from build123d import *

# Parameters (mm, degrees)
PAD_DEPTH    = 180
PAD001_DEPTH = 180


with BuildPart() as part:
    # Sketch → Pad (new body)
    with BuildSketch(Plane.XZ):
        Polygon((1.709151, 14), (0.847738, 14), (0.847738, 15), (2.609062, 15), (2.609062, 12.991093), (1, 11.170912), (1, 1.090989), (14, 1.090989), (14, 11.170912), (12.390938, 12.991093), (12.390938, 15), (14.152262, 15), (14.152262, 14), (13.290849, 14), (13.290849, 13.145577), (15, 11.212176), (15, 0), (0, 0), (0, 11.212176), (1.709151, 13.145577), align=None)
    extrude(amount=PAD_DEPTH)

    # Sketch001 → Pad001 (join)
    with BuildSketch(Plane.XZ):
        Polygon((1.670899, 13.98237), (0.833981, 13.98237), (0.833981, 15.0478), (14.219909, 15.0478), (14.219909, 13.970164), (13.277989, 13.970164), (13.277989, 13.140446), (14.96773, 13.140446), (14.96773, 15.855778), (0.035527, 15.855778), (0.035527, 13.198529), (1.670899, 13.198529), align=None)
    extrude(amount=PAD001_DEPTH)


solid = part.part
Work out the finished part from the listing and answer in its coordinate system (mm). A direction names the side the tool comes from. Give positions to 0.01 mm unless a question says otherwise; leave off trailing zeros. Order: outer loops, then holes, each group sorted by start corner. A loop starts at its lowest first (then second) coordinate and runs counter-clockwise, first axis right, second up. Notation, with made-up numbers: (18.5, 24) -> (50.5, 24) arc R6 cw to (50.5, 34) -> close; hole circle Ø3 at (12, 47.5). An arc over 180 degrees is marked (long way). Answer as a JSON object with one key per item and string values. Group by question number.
1. Section B-B on z = 7.5 is taken. Determine the outline of the cut face in (x, y).
2. Consider line 1 along X through (y, z) = (-63, 10); line 2 along Z through (x, y) = (5.75, -39); line 3 along X through (y, z) = (-80.5, 12.5). Determine where each line is inside the solid, lowest interval first. Write a range as [from, to].
3. Section A-A on x = 5 is taken. Determine the outline of the cut face in (y, z).
4. The mould has two halves that part along Y. Classify faces 3 (the flat face through (0.7, 0, 8)), 4 (the flat face through (14, -89, 6)), 5 (the flat face through (0.7, -180, 8)): released by +Y, released by -Y, zero draft, split by the parting line, or undercut.
5. Flat-ended cylindrical pins translate along their axes: pin 1 Ø3 at (y, z) = (-58.5, 14.5) entering from +X; pin 2 Ø1.5 at (x, z) = (11.5, 4) entering from +Y; pin 3 Ø1.2 at (y, z) = (-52.5, 14.5) entering from -X. Find the tip coordinate at first contact, or state that the pin passes through.
6. A tool of negligible diameter and unlimited length cuts with its end or side. For faces 1 (the flat face through (15, -89, 6)), 2 (the flat face through (1, -89, 6)), from which of +Z, -Z, +X, -X, +Y, -Y can it reach the whole face along a straight path? Write none if from no direction.
Result sheet:
{
 "1": {"outline": "(0, -180) -> (1, -180) -> (1, 0) -> (0, 0) -> close; (14, -180) -> (15, -180) -> (15, 0) -> (14, 0) -> close"},
 "2": {"line 1": "x = [0, 1], [14, 15]", "line 2": "z = [0, 1.09], [15.05, 15.86]", "line 3": "x = [1.14, 2.17], [12.83, 13.86]"},
 "3": {"outline": "(-180, 0) -> (0, 0) -> (0, 1.09) -> (-180, 1.09) -> close; (-180, 15.05) -> (0, 15.05) -> (0, 15.86) -> (-180, 15.86) -> close"},
 "4": {"face 3": "released by +Y", "face 4": "zero draft", "face 5": "released by -Y"},
 "5": {"pin 1": "stops at x = 14.97", "pin 2": "passes through", "pin 3": "stops at x = 0.04"},
 "6": {"face 1": "+Z, -Z, +X, +Y, -Y", "face 2": "+Y, -Y"}
}
